```python
from build123d import *

# Parameters (mm, degrees)
CROQUIS1_W              = 33.7
CROQUIS1_H              = 15.7
SALIENTE_EXTRUIR1_DEPTH = 5
CROQUIS2_W              = 31.7
CROQUIS2_H              = 13.7
SALIENTE_EXTRUIR2_DEPTH = 2
CORTAR_EXTRUIR1_DEPTH   = 10
CROQUIS4_W              = 33.7
CROQUIS4_H              = 15.7
SALIENTE_EXTRUIR3_DEPTH = 5
CROQUIS6_R              = 3
SALIENTE_EXTRUIR5_DEPTH = 4
SALIENTE_EXTRUIR6_DEPTH = 12
CROQUIS8_R              = 1.3
CORTAR_EXTRUIR2_DEPTH   = 6


with BuildPart() as part:
    # Croquis1 → Saliente-Extruir1 (new body)
    with BuildSketch(Plane(origin=(0, 0, 178), x_dir=(-1, 0, 0), z_dir=(0, 0, -1))):
        with Locations((13.350397628, -3.774933729)):
            Rectangle(CROQUIS1_W, CROQUIS1_H)
    extrude(amount=SALIENTE_EXTRUIR1_DEPTH)

    # Croquis2 → Saliente-Extruir2 (add)
    with BuildSketch(Plane.XY.offset(178)):
        with Locations((-13.350397628, -3.774933729)):
            Rectangle(CROQUIS2_W, CROQUIS2_H)
    extrude(amount=SALIENTE_EXTRUIR2_DEPTH)

    # Croquis3 → Cortar-Extruir1 (cut)
    with BuildSketch(Plane.XY.offset(180)):
        with BuildLine():
            Line((-25.250397628, 2.125066271), (-1.450397628, 2.125066271))
            ThreePointArc((-1.450397628, 2.125066271), (-0.319026778, 1.656437121), (0.149602372, 0.525066271))
            Line((0.149602372, 0.525066271), (0.149602372, -8.074933729))
            ThreePointArc((0.149602372, -8.074933729), (-0.319026778, -9.206304579), (-1.450397628, -9.674933729))
            Line((-1.450397628, -9.674933729), (-25.250397628, -9.674933729))
            ThreePointArc((-25.250397628, -9.674933729), (-26.381768478, -9.206304579), (-26.850397628, -8.074933729))
            Line((-26.850397628, -8.074933729), (-26.850397628, 0.525066271))
            ThreePointArc((-26.850397628, 0.525066271), (-26.381768478, 1.656437121), (-25.250397628, 2.125066271))
        make_face()
    extrude(amount=-CORTAR_EXTRUIR1_DEPTH, mode=Mode.SUBTRACT)

    # Croquis4 → Saliente-Extruir3 (add)
    with BuildSketch(Plane(origin=(0, 0, 173), x_dir=(-1, 0, 0), z_dir=(0, 0, -1))):
        with Locations((13.350397628, -3.774933729)):
            Rectangle(CROQUIS4_W, CROQUIS4_H)
        with BuildLine():
            Line((1.450397628, -9.674933729), (25.250397628, -9.674933729))
            ThreePointArc((25.250397628, -9.674933729), (26.381768478, -9.206304579), (26.850397628, -8.074933729))
            Line((26.850397628, -8.074933729), (26.850397628, 0.525066271))
            ThreePointArc((26.850397628, 0.525066271), (26.381768478, 1.656437121), (25.250397628, 2.125066271))
            Line((25.250397628, 2.125066271), (1.450397628, 2.125066271))
            ThreePointArc((1.450397628, 2.125066271), (0.319026778, 1.656437121), (-0.149602372, 0.525066271))
            Line((-0.149602372, 0.525066271), (-0.149602372, -8.074933729))
            ThreePointArc((-0.149602372, -8.074933729), (0.319026778, -9.206304579), (1.450397628, -9.674933729))
        make_face(mode=Mode.SUBTRACT)
    extrude(amount=SALIENTE_EXTRUIR3_DEPTH)

    # Croquis6 → Saliente-Extruir5 (add)
    with BuildSketch(Plane(origin=(0, 0, 168), x_dir=(-1, 0, 0), z_dir=(0, 0, -1))):
        with Locations((-3.499602372, -3.774933729)):
            Circle(CROQUIS6_R)
        with Locations((30.200397628, -3.774933729)):
            Circle(CROQUIS6_R)
    extrude(amount=-SALIENTE_EXTRUIR5_DEPTH)

    # Croquis7 → Saliente-Extruir6 (add)
    with BuildSketch(Plane(origin=(0, 0, 168), x_dir=(-1, 0, 0), z_dir=(0, 0, -1))):
        with BuildLine():
            Line((20.284128272, -9.674933729), (26.850397628, -6.079245942))
            Line((26.850397628, -6.079245942), (26.850397628, -8.074933729))
            ThreePointArc((26.850397628, -8.074933729), (26.381768478, -9.206304579), (25.250397628, -9.674933729))
            Line((25.250397628, -9.674933729), (20.284128272, -9.674933729))
        make_face()
    extrude(amount=-SALIENTE_EXTRUIR6_DEPTH)

    # Croquis8 → Cortar-Extruir2 (cut)
    with BuildSketch(Plane(origin=(0, 0, 168), x_dir=(-1, 0, 0), z_dir=(0, 0, -1))):
        with Locations((-3.499602372, -3.774933729)):
            Circle(CROQUIS8_R)
        with Locations((30.200397628, -3.774933729)):
            Circle(CROQUIS8_R)
    extrude(amount=-CORTAR_EXTRUIR2_DEPTH, mode=Mode.SUBTRACT)


solid = part.part
```
Verification items for the finished model (mm, model axes). A direction names the side the tool comes from. Coordinates: 2 decimals unless noted, no trailing zeros. Write each loop counter-clockwise with the first axis right and the second up, starting at its lowest first coordinate (ties: lowest second). Pieces come first, ordered by that corner, then holes. Notation, with made-up numbers: M 76,-21 L 103,-21 A21 cw 103,-1 Z; hole C 55.25,-15 d11. An arc over 180 degrees is marked long. Answer as a JSON object with one key per item and string values. Group by question number.
(1) Cross-section at A-A, the plane x = -7.5. Record the cut outline in (y, z).
(2) Tool access check on faces 5 (the face through (-11, -9.675, 174)), 6 (the face through (5, -4, 172)), 7 (the face through (-14, 3.075, 179)), 8 (the face through (-14, -10.625, 179)), 9 (the face through (-30.2, -3.9, 174.2)). Record the directions out of +Z, -Z, +X, -X, +Y, -Y that give a thin tool (end or side, any length) a straight path to the whole face; none if there is none.
(3) Material ranges on line 1 (Y direction, x = -10, z = 179); line 2 (X direction, y = -0.5, z = 170); line 3 (Y direction, x = -3, z = 174.5), recorded low to high.
(4) Cross-section at D-D, the plane x = -27.5. Record the cut outline in (y, z), and give its area (3 significant figures).
(5) Cross-section at B-B, the plane y = -1.75. Record the cut outline in (x, z), and give its area (3 significant figures).
(6) Gauge pin test, flat ends, axial feed: pin 1 (2 mm diameter, centred on y = -1.5, z = 174, fed in from +X); pin 2 (3 mm diameter, centred on y = -1.5, z = 171.5, fed in from -X); pin 3 (2 mm diameter, centred on y = -5.5, z = 178.5, fed in from -X). Record the tip position at first contact, or that the pin passes through.
(7) Cross-section at C-C, the plane z = 178.5. Record the cut outline in (x, y), and give its area (3 significant figures).
(8) Release check for a two-part mould opening along Y. For faces 1 (the face through (-30, -4, 174)), 2 (the face through (6.5, -3.7, 170)), 3 (the face through (-14, 2.125, 174)), 4 (the face through (-16, -10, 168)) record: +Y half, -Y half, draft (parallel to the pull), parting line (faces both ways), or undercut.
Reply:
{
 "1": {"outline": "M -11.62,168 L -9.67,168 L -9.67,180 L -10.62,180 L -10.62,178 L -11.62,178 Z; M 2.13,168 L 4.08,168 L 4.08,178 L 3.08,178 L 3.08,180 L 2.13,180 Z"},
 "2": {"face 5": "+Z, -Z", "face 6": "+Z, +X, +Y, -Y", "face 7": "+Z, +X, -X, +Y", "face 8": "+Z, +X, -X, -Y", "face 9": "+Z, -X"},
 "3": {"line 1": "-10.62 to -9.67, 2.13 to 3.08", "line 2": "-30.2 to -26.85, 0.15 to 3.5", "line 3": "-11.62 to -9.67, 2.13 to 4.08"},
 "4": {"outline": "M -11.62,168 L 4.08,168 L 4.08,178 L 3.08,178 L 3.08,180 L -10.62,180 L -10.62,178 L -11.62,178 Z", "area": "184 mm²"},
 "5": {"outline": "M -32.41,168 L -26.85,168 L -26.85,180 L -29.2,180 L -29.2,178 L -30.2,178 L -30.2,172 L -32.41,172 Z; M 0.15,168 L 5.71,168 L 5.71,172 L 3.5,172 L 3.5,178 L 2.5,178 L 2.5,180 L 0.15,180 Z", "area": "94.1 mm²"},
 "6": {"pin 1": "x = 3.5", "pin 2": "x = -33.1", "pin 3": "x = -30.2"},
 "7": {"outline": "M -29.2,-10.62 L 2.5,-10.62 L 2.5,3.08 L -29.2,3.08 Z; hole M -26.85,-6.08 L -20.28,-9.67 L -1.45,-9.67 A1.6 ccw 0.15,-8.07 L 0.15,0.53 A1.6 ccw -1.45,2.13 L -25.25,2.13 A1.6 ccw -26.85,0.53 Z", "area": "129 mm²"},
 "8": {"face 1": "undercut", "face 2": "parting line", "face 3": "undercut", "face 4": "draft"}
}
